from build123d import *

# Parameters (mm, degrees)
F1_DEPTH = 6.1341
F3_D     = 4.2164
F5_DEPTH = 6.1341
F7_D     = 4.2164


with BuildPart() as f1:
    # F0 (on Top) → F1 (new body)
    with BuildSketch(Plane.XY):
        Polygon((-30.502569, 5.842), (-10.191964, -29.337), (10.191964, -29.337), (30.502569, 5.842), (20.310605, 23.495), (-20.310605, 23.495), align=None)
    extrude(amount=F1_DEPTH)

    # F3 (through all)
    with Locations(Plane.XY.offset(6.1341)):
        with Locations((-17.964254, 19.431), (-25.809866, 5.842), (-7.845613, -25.273), (7.845613, -25.273), (25.809866, 5.842), (17.964254, 19.431)):
            Hole(F3_D / 2)

    # F4 (on face) → F5 (cut, through all)
    with BuildSketch(Plane.XY.offset(6.1341)):
        with BuildLine():
            Line((-6.5405, 23.495), (-6.5405, 0))
            ThreePointArc((-6.5405, 0), (0, -6.5405), (6.5405, 0))
            Line((6.5405, 0), (6.5405, 23.495))
            Line((6.5405, 23.495), (-6.5405, 23.495))
        make_face()
    extrude(amount=-F5_DEPTH, mode=Mode.SUBTRACT)

    # F7 (through all)
    with Locations(Plane.XY.offset(6.1341)):
        with Locations((-10.795, 11.43), (10.795, 11.43)):
            Hole(F7_D / 2)


solid = f1.part
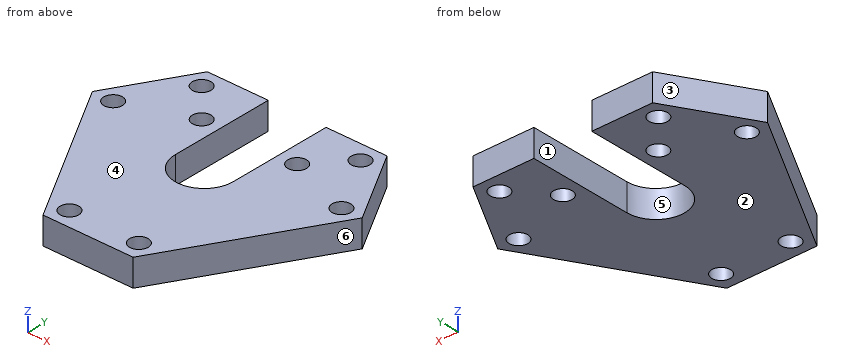
Design review of the part built by this model. Coordinates are the model's own, in mm. Face numbers are marked on the shaded views. A direction names the side the tool comes from. Round coordinates to 2 decimals unless told otherwise and drop trailing zeros. Write each loop counter-clockwise with the first axis right and the second up, starting at its lowest first coordinate (ties: lowest second). Pieces come first, ordered by that corner, then holes. Notation, with made-up numbers: (12.25, -21) -> (26.25, -21) arc R21 ccw to (26.25, 9) -> close; hole circle Ø11 at (-19, 87). An arc over 180 degrees is marked (long way). One line per question, with ' | ' between items.
(1) Take a section at D-D, the plane x = 0. State the section outline as (y, z) points, and give its area (3 significant figures).
Result sheet:
outline: (-29.34, 0) -> (-6.54, 0) -> (-6.54, 6.13) -> (-29.34, 6.13) -> close | area: 140 mm2
(2) Machinability: for the marked faces 1 and 2, which of the approach directions +Z, -Z, +X, -X, +Y, -Y give a long, thin tool a straight path to every point of the face, cutting with its end or side? Answer none if there is none.
Result sheet:
face 1: +Z, -Z, +Y | face 2: -Z, +X, -X, +Y, -Y
(3) Wall thickness on line 1 (Y direction, x = 9, z = 3) (3 decimals); line 2 (Y direction, x = -7.5, z = 0.5) (3 decimals); line 3 (X direction, y = 0, z = 2.5): over which ranges is each line inside the solid? List them lowest first. Write a range as [from, to].
Result sheet:
line 1: [-29.337, -27.037], [-23.509, 10.324], [12.536, 23.495] | line 2: [-29.337, -27.353], [-23.193, 23.495] | line 3: [-27.13, -6.54], [6.54, 27.13]
(4) Draft analysis for pull direction X (two halves, no side actions). For the marked faces 3, 4, 5 and 6, state which applies: released by +X, released by -X, zero draft, split by the parting line, or undercut.
Result sheet:
face 3: released by -X | face 4: zero draft | face 5: undercut | face 6: released by +X
(5) Take a section at A-A, the plane y = 11.43. State the section outline as (x, z) points.
Result sheet:
outline: (-27.28, 0) -> (-12.9, 0) -> (-12.9, 6.13) -> (-27.28, 6.13) -> close; (-8.69, 0) -> (-6.54, 0) -> (-6.54, 6.13) -> (-8.69, 6.13) -> close; (6.54, 0) -> (8.69, 0) -> (8.69, 6.13) -> (6.54, 6.13) -> close; (12.9, 0) -> (27.28, 0) -> (27.28, 6.13) -> (12.9, 6.13) -> close
(6) Take a section at C-C, the plane y = -4. State the section outline as (x, z) points, and give its area (3 significant figures).
Result sheet:
outline: (-24.82, 0) -> (-5.17, 0) -> (-5.17, 6.13) -> (-24.82, 6.13) -> close; (5.17, 0) -> (24.82, 0) -> (24.82, 6.13) -> (5.17, 6.13) -> close | area: 241 mm2
(7) Take a section at B-B, the plane z = 3. State how many separate pieces and enclosed holes the cut face has, and give its area (3 significant figures).
Result sheet:
separate pieces: 1 | enclosed holes: 8 | area: 1,840 mm2
(8) Insertion check: P1, Ø1, axis at x = -1.5, z = 2.5, coming from the +Y side; P2, Ø3, axis at y = 10.5, z = 3.5, coming from the +X side; P3, Ø2, axis at y = -12.5, z = 1, coming from the +X side. Each pin has a flat end and moves straight along its axis. Give the tip position at first contact, or say it passes through.
Result sheet:
P1: y = -6.23 | P2: x = 28.68 | P3: x = 20.49
